from build123d import *
from build123d import SkipClean  # not in build123d's __all__

# Parameters (mm, degrees)
F1_DEPTH = 7
F3_DEPTH = 18
F4_DEPTH = 4
F6_DEPTH = 4
F7_R     = 1.5
F8_DEPTH = 3.5


with BuildPart() as f1:
    # F0 (on Top) → F1 (new body)
    with BuildSketch(Plane.XY):
        Polygon((-8.6863613641, -3.3171127737), (0.3136386359, -3.3171127737), (9.3136386359, -3.3171127737), (9.3136386359, 0.1828872263), (9.3136386359, 9.1828872263), (5.3136386359, 9.1828872263), (5.3136386359, 0.1828872263), (-4.6863613641, 0.1828872263), (-4.6863613641, 9.1828872263), (-8.6863613641, 9.1828872263), (-8.6863613641, 0.1828872263), align=None)
    extrude(amount=F1_DEPTH)

    # F2 (on face) → F3 (cut, through all)
    with BuildSketch(Plane(origin=(-8.6863613641, 0, 0), x_dir=(0, -1, 0), z_dir=(-1, 0, 0))):
        with BuildLine():
            Line((-9.1828872263, 5.5), (-9.1828872263, 1.5))
            ThreePointArc((-9.1828872263, 1.5), (-7.768673664, 2.0857864376), (-7.1828872263, 3.5))
            ThreePointArc((-7.1828872263, 3.5), (-7.768673664, 4.9142135624), (-9.1828872263, 5.5))
        make_face()
    extrude(amount=-F3_DEPTH, mode=Mode.SUBTRACT)

    # F2 (on face) → F4 (join, through all)
    with BuildSketch(Plane(origin=(-8.6863613641, 0, 0), x_dir=(0, -1, 0), z_dir=(-1, 0, 0))):
        with BuildLine():
            ThreePointArc((-9.1828872263, 7), (-12.6828872263, 3.5), (-9.1828872263, 0))
            Line((-9.1828872263, 0), (-9.1828872263, 1.5))
            ThreePointArc((-9.1828872263, 1.5), (-11.1828872263, 3.5), (-9.1828872263, 5.5))
            Line((-9.1828872263, 5.5), (-9.1828872263, 7))
        make_face()
    with SkipClean():  # cleaning this boolean's faces spoils the solid; the shape is the same uncleaned
        extrude(amount=-F4_DEPTH)

    # F5 (on face) → F6 (join, through all)
    with BuildSketch(Plane.YZ.offset(9.3136386359)):
        with BuildLine():
            ThreePointArc((9.1828872263, 1.5), (7.1828872263, 3.5), (9.1828872263, 5.5))
            Line((9.1828872263, 5.5), (9.1828872263, 7))
            ThreePointArc((9.1828872263, 7), (5.6828872263, 3.5), (9.1828872263, 0))
            Line((9.1828872263, 0), (9.1828872263, 1.5))
        make_face()
        with BuildLine():
            Line((9.1828872263, 7), (9.1828872263, 5.5))
            ThreePointArc((9.1828872263, 5.5), (10.5971007887, 4.9142135624), (11.1828872263, 3.5))
            ThreePointArc((11.1828872263, 3.5), (10.5971007887, 2.0857864376), (9.1828872263, 1.5))
            Line((9.1828872263, 1.5), (9.1828872263, 0))
            ThreePointArc((9.1828872263, 0), (11.6577609605, 1.0251262658), (12.6828872263, 3.5))
            ThreePointArc((12.6828872263, 3.5), (11.6577609605, 5.9748737342), (9.1828872263, 7))
        make_face()
        with BuildLine():
            ThreePointArc((9.1828872263, 0), (5.6828872263, 3.5), (9.1828872263, 7))
            Line((9.1828872263, 7), (-3.3171127737, 7))
            Line((-3.3171127737, 7), (-3.3171127737, 0))
            Line((-3.3171127737, 0), (9.1828872263, 0))
        make_face()
    extrude(amount=-F6_DEPTH)

    # F7 (on face) → F8 (cut, through all)
    with BuildSketch(Plane.XZ.offset(3.3171127737)):
        with Locations((-2.5, 3.5)):
            Circle(F7_R)
        with Locations((2.5, 3.5)):
            Circle(F7_R)
    extrude(amount=-F8_DEPTH, mode=Mode.SUBTRACT)


solid = f1.part
Here's how the part is built. I have some questions about the finished solid (model axes, mm). A direction names the side the tool comes from. Round coordinates to 2 decimals unless told otherwise and drop trailing zeros. Write each loop counter-clockwise with the first axis right and the second up, starting at its lowest first coordinate (ties: lowest second). Pieces come first, ordered by that corner, then holes.
1. Suppose I cut it at D-D (y = -1). List the corners of the cut face in (x, z) for me.
2. Suppose I cut it at B-B (y = 3.5). List the corners of the cut face in (x, z) for me, and give its area (3 significant figures).
3. For faces 5 (the flat face through (5.314, 5, 3)), 6 (the flat face through (0, -1, 0)), which set-ups out of +Z, -Z, +X, -X, +Y, -Y let a thin tool reach every point of the face, with its end or its side?
4. I need wall thicknesses on L1, parallel to Z at x = -2.5, y = -1.95; L2, parallel to Z at x = -5.25, y = 9.25; L3, parallel to Y at x = -2.25, z = 1.5. Which ranges of each line are inside material? Lowest first, please.
5. Suppose I cut it at C-C (z = 2.75). List the corners of the cut face in (x, y) for me, and give its area (3 significant figures).
6. If we mould it in two halves opening along X, with no side actions, what happens to faces 1 (the flat face through (9.314, 5, 3)), 2 (the flat face through (0, 0.183, 3)), 3 (the flat face through (-8.686, 3, 3)), 4 (the cylindrical face through (-1.07, -1.59, 3.95))? For each: released by +X, released by -X, zero draft, split by the parting line, or undercut.
7. Will these pins go through, and if not, where does the flat tip stop? pin 1 Ø4 at (x, z) = (3, 1.5) entering from +Y; pin 2 Ø1 at (y, z) = (8, 3.5) entering from -X.
8. Suppose I cut it at A-A (x = -2.5). List the corners of the cut face in (y, z) for me.
Answer sheet:
1. outline: (-8.69, 0) - (9.31, 0) - (9.31, 7) - (-8.69, 7) - close; hole circle Ø3 at (-2.5, 3.5); hole circle Ø3 at (2.5, 3.5)
2. outline: (-8.69, 0) - (-4.69, 0) - (-4.69, 7) - (-8.69, 7) - close; (5.31, 0) - (9.31, 0) - (9.31, 7) - (5.31, 7) - close
2. area: 56.0 mm2
3. face 5: +Z, -Z, +Y
3. face 6: -Z, +X, -X, +Y, -Y
4. L1: z = 0 to 2, 5 to 7
4. L2: z = 0 to 1.5, 5.5 to 7
4. L3: y = -3.32 to 0.18
5. outline: (-8.69, -3.32) - (-3.8, -3.32) - (-3.8, 0.18) - (-4.69, 0.18) - (-4.69, 7.33) - (-8.69, 7.33) - close; (-8.69, 11.04) - (-4.69, 11.04) - (-4.69, 12.6) - (-8.69, 12.6) - close; (-1.2, -3.32) - (1.2, -3.32) - (1.2, 0.18) - (-1.2, 0.18) - close; (3.8, -3.32) - (9.31, -3.32) - (9.31, 7.33) - (5.31, 7.33) - (5.31, 0.18) - (3.8, 0.18) - close; (5.31, 11.04) - (9.31, 11.04) - (9.31, 12.6) - (5.31, 12.6) - close
5. area: 114 mm2
6. face 1: released by +X
6. face 2: undercut
6. face 3: released by -X
6. face 4: undercut
7. pin 1: stops at y = 0.18
7. pin 2: passes through
8. outline: (-3.32, 0) - (0.18, 0) - (0.18, 2) - (-3.32, 2) - close; (-3.32, 5) - (0.18, 5) - (0.18, 7) - (-3.32, 7) - close
